Build history of the part. All positions in model axes, mm. Round coordinates to 2 decimals unless told otherwise and drop trailing zeros. Loops run counter-clockwise (first coordinate to the right, second up) from the corner with the lowest first, then second, coordinate; pieces in that order, holes last. Notation, with made-up numbers: (-27.75, -18) -> (-0.75, -18) arc R30 cw to (-0.75, 7) -> close; hole circle Ø2 at (0, 79.5). An arc over 180 degrees is marked (long way). Put each result on its own line as item: value. Start each with the question number.
Item 1: Cut at D-D, the plane x = 8.25. List the corners of the cut face in (y, z).
Item 2: Cut at C-C, the plane z = 2.5. List the corners of the cut face in (x, y), plus the area to 3 significant figures.
Item 3: Cut at B-B, the plane z = -2.25. List the corners of the cut face in (x, y), plus the area to 3 significant figures.
Item 4: Cut at A-A, the plane y = 6.5. List the corners of the cut face in (x, z), plus the area to 3 significant figures.
Item 5: Pull direction X, two halves, no side cores. Call faces 1 (the cylindrical face through (11.297, 11.859, -0.056)), 2 (the flat face through (0, 0, 0)), 3 (the cylindrical face through (-0.1, 6.6, -0.9)): +X half, -X half, draft (parallel to the pull), parting line (faces both ways), or undercut.
Item 6: Drill centre lines: probe 1 along X at (y, z) = (5.5, 3.25); probe 2 along Y at (x, z) = (9, 1.5); probe 3 along Y at (x, z) = (-7.25, 2). Where is each one in solid material? Low to high. Write a range as [from, to].
Item 7: Flat gauge pin, fed straight in: pin 1 Ø6 at (x, y) = (2.5, 11) entering from -Z. Where does the tip first touch, or does it go through?
```python
from build123d import *

# Parameters (mm, degrees)
SKETCH1_W           = 25
SKETCH1_H           = 8
BOSS_EXTRUDE1_DEPTH = 13
SKETCH2_R           = 4.1
CUT_EXTRUDE1_DEPTH  = 19.472953202
SKETCH3_R           = 1.65
CUT_EXTRUDE2_DEPTH  = 10
FILLET2_R           = 4


with BuildPart() as part:
    # Sketch1 → Boss-Extrude1 (new body)
    with BuildSketch(Plane(origin=(0, 0, 0), x_dir=(1, 0, 0), z_dir=(0, 1, 0))):
        Rectangle(SKETCH1_W, SKETCH1_H)
    extrude(amount=BOSS_EXTRUDE1_DEPTH)

    # Sketch2 → Cut-Extrude1 (cut, through all)
    with BuildSketch(Plane(origin=(0, 13, 0), x_dir=(1, 0, 0), z_dir=(0, 1, 0))):
        with Locations((0, 5)):
            Circle(SKETCH2_R)
    extrude(amount=-CUT_EXTRUDE1_DEPTH, mode=Mode.SUBTRACT)

    # Sketch3 → Cut-Extrude2 (cut)
    with BuildSketch(Plane(origin=(0, 0, -4), x_dir=(-1, 0, 0), z_dir=(0, 0, -1))):
        with Locations((8.238089535, 6.5)):
            Circle(SKETCH3_R)
        with Locations((-8.238089535, 6.5)):
            Circle(SKETCH3_R)
    extrude(amount=-CUT_EXTRUDE2_DEPTH, mode=Mode.SUBTRACT)

    # Fillet2
    fillet2_edges = [part.edges().sort_by_distance(p)[0] for p in [
        (-12.5, 13, 0),
        (12.5, 13, 0),
        (-12.5, 0, 0),
        (12.5, 0, 0),
    ]]
    fillet(fillet2_edges, radius=FILLET2_R)


solid = part.part
```
Reply:
1. outline: (0, -4) -> (4.85, -4) -> (4.85, 4) -> (0, 4) -> close; (8.15, -4) -> (13, -4) -> (13, 4) -> (8.15, 4) -> close
2. outline: (-12.5, 4) arc R4 ccw to (-8.5, 0) -> (8.5, 0) arc R4 ccw to (12.5, 4) -> (12.5, 9) arc R4 ccw to (8.5, 13) -> (-8.5, 13) arc R4 ccw to (-12.5, 9) -> close; hole circle Ø3.3 at (-8.24, 6.5); hole circle Ø3.3 at (8.24, 6.5)
2. area: 294 mm^2
3. outline: (-12.5, 4) arc R4 ccw to (-8.5, 0) -> (-3.04, 0) -> (-3.04, 13) -> (-8.5, 13) arc R4 ccw to (-12.5, 9) -> close; (3.04, 0) -> (8.5, 0) arc R4 ccw to (12.5, 4) -> (12.5, 9) arc R4 ccw to (8.5, 13) -> (3.04, 13) -> close; hole circle Ø3.3 at (-8.24, 6.5); hole circle Ø3.3 at (8.24, 6.5)
3. area: 215 mm^2
4. outline: (-12.5, -4) -> (-9.89, -4) -> (-9.89, 4) -> (-12.5, 4) -> close; (-6.59, -4) -> (-3.98, -4) arc R4.1 cw to (3.98, -4) -> (6.59, -4) -> (6.59, 4) -> (-6.59, 4) -> close; (9.89, -4) -> (12.5, -4) -> (12.5, 4) -> (9.89, 4) -> close
4. area: 129 mm^2
5. face 1: +X half
5. face 2: draft
5. face 3: undercut
6. probe 1: x = [-12.5, -9.55], [-6.93, 6.93], [9.55, 12.5]
6. probe 2: y = [0.03, 5.04], [7.96, 12.97]
6. probe 3: y = [0, 5.18], [7.82, 13]
7. pin 1: stops at z = -4
